Model file for the job. Use its own axes, mm. A direction names the side the tool comes from. Round coordinates to 2 decimals unless told otherwise and drop trailing zeros. Order: outer loops, then holes, each group sorted by start corner. A loop starts at its lowest first (then second) coordinate and runs counter-clockwise, first axis right, second up. Notation, with made-up numbers: (3, -24.75) - (42, -24.75) arc R23 cw to (42, -12.75) - close; hole circle Ø7 at (-34, 75.5). An arc over 180 degrees is marked (long way). Put each result on its own line as item: value. Start each with the question number.
Item 1: Mould opens along X. For faces 3 (the face through (-0.54, 0.04, 45.06)), 4 (the face through (-0.54, -17.44, -44.96)), 5 (the face through (0, -27.5, -45)), 6 (the face through (-15, -2, -7)) say: pulls with the +X half, pulls with the -X half, needs draft (parallel to the pull), parting line crosses it, or undercut.
Item 2: Which spindle directions (+Z, -Z, +X, -X, +Y, -Y) get a long thin tool onto all of the face, cutting with end or side? Do faces 1 (the face through (0, -12, -42.5)), 2 (the face through (15, -2, -7)). Say none if no direction does.
Item 3: Saw through at B-B on y = -15. List the corners of the cut face in (x, z).
Item 4: Saw through at D-D on z = -25.5. List the corners of the cut face in (x, y), plus the area to 3 significant figures.
Item 5: Saw through at C-C on x = 9.5. List the corners of the cut face in (y, z).
Item 6: Pin check, flat tips, straight feed: pin 1 Ø15 at (x, z) = (-7, -4) entering from -Y; pin 2 Ø4.5 at (x, y) = (0, -15) entering from -Z; pin 3 Ø12 at (x, y) = (6, -23) entering from +Z. Stop position of each tip, or through.
Item 7: Saw through at A-A on x = 0. List the corners of the cut face in (y, z).
Item 8: Probe probe 1 along Y at (x, z) = (0, -44.95); probe 2 along Z at (x, y) = (0, 0.8); probe 3 along Z at (x, y) = (0.75, -6). List the from-to ranges inside material, lowest first.
```python
from build123d import *

# Parameters (mm, degrees)
F0_R     = 2.5
F1_DEPTH = 2.5
F2_W     = 30
F2_H     = 5
F3_DEPTH = 25
F4_R     = 2.5
F5_DEPTH = 5


with BuildPart() as f1:
    # F0 (on Front) → F1 (new body, symmetric)
    with BuildSketch(Plane.XZ):
        with BuildLine():
            Line((-15, 47.5), (-15, -47.5))
            Line((-15, -47.5), (15, -47.5))
            Line((15, -47.5), (15, 47.5))
            ThreePointArc((15, 47.5), (0, 62.5), (-15, 47.5))
        make_face()
        with Locations((0, 47.5)):
            Circle(F0_R, mode=Mode.SUBTRACT)
    extrude(amount=F1_DEPTH, both=True)

    # F2 (on face) → F3 (join)
    with BuildSketch(Plane.XZ.offset(2.5)):
        with Locations((0, -45)):
            Rectangle(F2_W, F2_H)
    extrude(amount=F3_DEPTH)

    # F4 (on face) → F5 (cut, through all)
    with BuildSketch(Plane.XY.offset(-42.5)):
        with Locations((0, -15)):
            Circle(F4_R)
    extrude(amount=-F5_DEPTH, mode=Mode.SUBTRACT)


solid = f1.part
```
Results found:
1. face 3: undercut
1. face 4: undercut
1. face 5: needs draft
1. face 6: pulls with the -X half
2. face 1: +Z, +X, -X, -Y
2. face 2: +Z, -Z, +X, +Y, -Y
3. outline: (-15, -47.5) - (-2.5, -47.5) - (-2.5, -42.5) - (-15, -42.5) - close; (2.5, -47.5) - (15, -47.5) - (15, -42.5) - (2.5, -42.5) - close
4. outline: (-15, -2.5) - (15, -2.5) - (15, 2.5) - (-15, 2.5) - close
4. area: 150 mm²
5. outline: (-27.5, -47.5) - (2.5, -47.5) - (2.5, 59.11) - (-2.5, 59.11) - (-2.5, -42.5) - (-27.5, -42.5) - close
6. pin 1: stops at y = -2.5
6. pin 2: passes through
6. pin 3: stops at z = -42.5
7. outline: (-27.5, -47.5) - (-17.5, -47.5) - (-17.5, -42.5) - (-27.5, -42.5) - close; (-12.5, -47.5) - (2.5, -47.5) - (2.5, 45) - (-2.5, 45) - (-2.5, -42.5) - (-12.5, -42.5) - close; (-2.5, 50) - (2.5, 50) - (2.5, 62.5) - (-2.5, 62.5) - close
8. probe 1: y = -27.5 to -17.5, -12.5 to 2.5
8. probe 2: z = -47.5 to 45, 50 to 62.5
8. probe 3: z = -47.5 to -42.5
